Autodesk Inventor part; units mm, degrees
ref_plane "YZ Plane" through (0, 0, 0) normal (1, 0, 0) x (0, 1, 0)
ref_plane "XZ Plane" through (0, 0, 0) normal (0, 1, 0) x (-1, 0, 0)
ref_plane "XY Plane" through (0, 0, 0) normal (0, 0, 1) x (1, 0, 0)
sketch "Эскиз1" plane through (0, 0, 0) normal (0, 0, 1) x (1, 0, 0)
  circle A0 centre (0, 0) radius 2
  line L0 (-7.5, -14.5) -> (7.5, -14.5)
  line L1 (7.5, -14.5) -> (7.5, 0)
  line L2 (7.5, 0) -> (-7.5, 0) construction
  line L3 (-7.5, 0) -> (-7.5, -14.5)
  line L4 (0, -18.7) -> (0, 10.7) construction
  circle A1 centre (0, 0) radius 6.5 construction
  line L5 (-7.5, 0) -> (-4, 5)
  line L6 (-4, 5) -> (4, 5)
  line L7 (4, 5) -> (7.5, 0)
  point P0 (0, 5)
  point P1 (0, -14.5)
  dimension "d0" = 4
  dimension "d6" = 13
  dimension "d8" = 8
  dimension "d11" = 15
  dimension "d12" = 5
  dimension "d13" = 14.5
extrude "Выдавливание1" add sketch "Эскиз1" along normal blind 6
fillet "Сопряжение1" radius 7 4 edges at (-7.5, 0, 3) (-4, 5, 3) (4, 5, 3) (7.5, 0, 3)
properties part number "Крепление шкива"
Geometry: final body of the model. Coordinates: model frame, mm. Round coordinates to 2 decimals unless told otherwise and drop trailing zeros. Order: outer loops, then holes, each group sorted by start corner. A loop starts at its lowest first (then second) coordinate and runs counter-clockwise, first axis right, second up. Notation, with made-up numbers: (45.5, -23) - (98.5, -23) arc R21 cw to (98.5, -3) - close; hole circle Ø8 at (-8, 41). An arc over 180 degrees is marked (long way). Write item = value, one per line. Start each with the question number.
Q1. Pull-direction query (Y, two-part tool) for faces 1 (the cylindrical face through (0, 2, 3)), 2 (the flat face through (-7.5, -8, 3)), 3 (the cylindrical face through (-7.167, -0.074, 3.042)), 4 (the flat face through (0, -14.5, 3)); classes: +Y half, -Y half, draft (parallel to the pull), parting line (faces both ways), or undercut.
Q2. Cut plane B-B on z = 5.25. Return the cut outline in (x, y), and give its area (3 significant figures).
Q3. Cut plane C-C on y = -0.5. Return the cut outline in (x, z), and give its area (3 significant figures).
Q4. Ray query, line 1 (Y direction, x = 0, z = 3.15); line 2 (X direction, y = 1.25, z = 1.6); line 3 (Y direction, x = -0.5, z = 1.45). Return the intervals inside material, ascending. Write a range as from..to.
Q5. Cut plane D-D on y = 3. Return the cut outline in (x, z).
Q6. Cut plane A-A on x = 0. Return the cut outline in (y, z).
Outcome:
q1.face_1 = undercut
q1.face_2 = draft
q1.face_3 = +Y half
q1.face_4 = -Y half
q2.outline = (-7.5, -14.5) - (7.5, -14.5) - (7.5, -2.21) arc R7 ccw to (6.23, 1.81) - (6.09, 2.01) arc R7 ccw to (0.36, 5) - (-0.36, 5) arc R7 ccw to (-6.09, 2.01) - (-6.23, 1.81) arc R7 ccw to (-7.5, -2.21) - close; hole circle Ø4 at (0, 0)
q2.area = 257 mm^2
q3.outline = (-7.29, 0) - (-1.94, 0) - (-1.94, 6) - (-7.29, 6) - close; (1.94, 0) - (7.29, 0) - (7.29, 6) - (1.94, 6) - close
q3.area = 64.2 mm^2
q4.line_1 = -14.5..-2, 2..5
q4.line_2 = -6.59..-1.56, 1.56..6.59
q4.line_3 = -14.5..-1.94, 1.94..5
q5.outline = (-5.25, 0) - (5.25, 0) - (5.25, 6) - (-5.25, 6) - close
q6.outline = (-14.5, 0) - (-2, 0) - (-2, 6) - (-14.5, 6) - close; (2, 0) - (5, 0) - (5, 6) - (2, 6) - close
